Could you check a few things on this drawing? It's one solid part, dimensions in mm from its lowest x, y, z. A direction names the side the tool comes from. Give positions to 0.01 mm unless a question says otherwise; leave off trailing zeros. Loops run counter-clockwise (first coordinate to the right, second up) from the corner with the lowest first, then second, coordinate; pieces in that order, holes last. Notation, with made-up numbers: M 59.5,45.25 L 78.5,45.25 A14 ccw 78.5,56.25 Z; hole C 8,57.25 d6. An arc over 180 degrees is marked long. Return JSON: item names as keys, results as strings. Group by question number.
1. If we section it at B-B (z = 2.8): Write out the boundary of the cut face in (x, y).
2. If we mould it in two halves opening along Y, with no side actions, what happens to the marked faces 1, 2, 3 and 4? For each: +Y half, -Y half, draft (parallel to the pull), parting line (faces both ways), or undercut.
3. If we section it at C-C (x = 8): Write out the boundary of the cut face in (y, z), plus the area to 3 significant figures.
4. For the marked faces 5 and 6, which set-ups out of +Z, -Z, +X, -X, +Y, -Y let a thin tool reach every point of the face, with its end or its side?
5. Please list where these lines run through material, in increasing order: line 1 (X direction, y = 3, z = 1.45); line 2 (Y direction, x = 3, z = 2.05); line 3 (Y direction, x = 8.25, z = 0.8).
6. If we section it at A-A (x = 12.25): Write out the boundary of the cut face in (y, z).
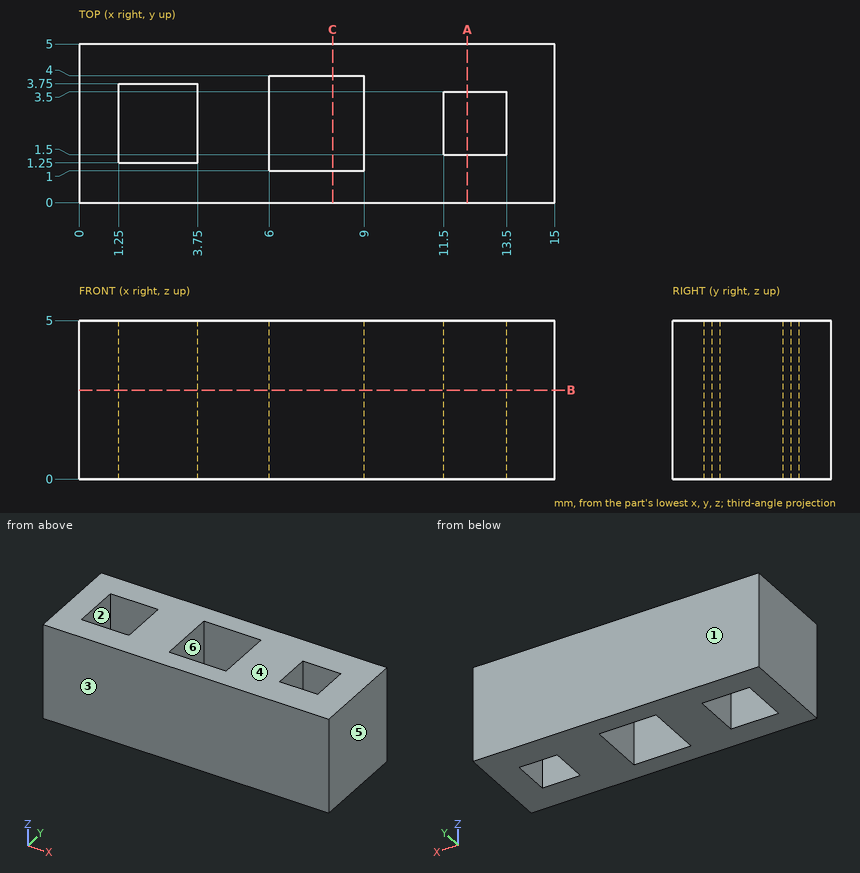
Answer:
{
 "1": {"outline": "M 0,0 L 15,0 L 15,5 L 0,5 Z; hole M 1.25,1.25 L 3.75,1.25 L 3.75,3.75 L 1.25,3.75 Z; hole M 6,1 L 9,1 L 9,4 L 6,4 Z; hole M 11.5,1.5 L 13.5,1.5 L 13.5,3.5 L 11.5,3.5 Z"},
 "2": {"face 1": "+Y half", "face 2": "undercut", "face 3": "-Y half", "face 4": "draft"},
 "3": {"outline": "M 0,0 L 1,0 L 1,5 L 0,5 Z; M 4,0 L 5,0 L 5,5 L 4,5 Z", "area": "10.0 mm²"},
 "4": {"face 5": "+Z, -Z, +X, +Y, -Y", "face 6": "+Z, -Z"},
 "5": {"line 1": "x = 0 to 1.25, 3.75 to 6, 9 to 11.5, 13.5 to 15", "line 2": "y = 0 to 1.25, 3.75 to 5", "line 3": "y = 0 to 1, 4 to 5"},
 "6": {"outline": "M 0,0 L 1.5,0 L 1.5,5 L 0,5 Z; M 3.5,0 L 5,0 L 5,5 L 3.5,5 Z"}
}
